```python
from build123d import *

# Parameters (mm, degrees)
F1_DEPTH = 50.8
F2_SIZE  = 5.08
F3_W     = 6.35
F3_H     = 6.35
F4_DEPTH = 38.1


with BuildPart() as f1:
    # F0 (on Front) → F1 (new body)
    with BuildSketch(Plane.XZ):
        Polygon((12.496759, 6.899342), (0.273374, 14.272182), (-12.223385, 7.37284), (-12.496759, -6.899342), (-0.273374, -14.272182), (12.223385, -7.37284), align=None)
    extrude(amount=F1_DEPTH)

    # F2
    f2_edges = [f1.edges().sort_by_distance(p)[0] for p in [
        (6.385067, 0, 10.585762),
        (12.360072, 0, -0.236749),
        (5.975005, 0, -10.822511),
        (-6.385067, 0, -10.585762),
        (-12.360072, 0, 0.236749),
        (-5.975005, 0, 10.822511),
    ]]
    chamfer(f2_edges, length=F2_SIZE)

    # F3 (on face) → F4 (cut)
    with BuildSketch(Plane(origin=(0, 0, 0), x_dir=(-1, 0, 0), z_dir=(0, 1, 0))):
        Rectangle(F3_W, F3_H)
    extrude(amount=-F4_DEPTH, mode=Mode.SUBTRACT)


solid = f1.part
```
The model under review builds one solid part; all positions refer to its coordinate system, in mm. A direction names the side the tool comes from. Coordinates: 2 decimals unless noted, no trailing zeros. Order: outer loops, then holes, each group sorted by start corner. A loop starts at its lowest first (then second) coordinate and runs counter-clockwise, first axis right, second up. Notation, with made-up numbers: (16.5, -39) -> (65.5, -39) arc R24 ccw to (65.5, -27) -> close; hole circle Ø2 at (74, 72). An arc over 180 degrees is marked (long way). Answer in a Markdown table with one row per item. Add a question column.
Item 1: To check wall thickness, follow probe 1 along Y at (x, z) = (-2.5, -2); probe 2 along Z at (x, y) = (0.5, -22.5) (3 decimals); probe 3 along Z at (x, y) = (-1.5, -25) (3 decimals). State the ranges of each line that lie inside material, in increasing order.
Item 2: Mouldability with a two-part tool opening along Z and no side actions: class faces 1 (the flat face through (3.175, -19, 0)), 2 (the flat face through (-3.175, -19, 0)), 3 (the flat face through (-5.89, -27.62, 10.87)), 4 (the flat face through (-6.471, -27.62, -10.534)) as +Z half, -Z half, draft (parallel to the pull), parting line (faces both ways), or undercut.
Item 3: We need section A-A on y = -29. Write out the cut boundary in (x, z) (3 decimals).
Item 4: Clearance check with flat-ended pins moving along their axes: pin 1 (3 mm diameter, centred on x = -0.5, y = -28, fed in from -Z); pin 2 (1.5 mm diameter, centred on y = -43.5, z = 10.5, fed in from +X); pin 3 (7 mm diameter, centred on y = -18.5, z = 0, fed in from +X); pin 4 (3 mm diameter, centred on x = 3, y = -31.5, fed in from +Z). State where each tip first meets the part, or that it passes through.
Item 5: Machinability: for faces 5 (the flat face through (0, -50.8, 0)), 6 (the flat face through (0, -38.1, 0)), which of the approach directions +Z, -Z, +X, -X, +Y, -Y give a long, thin tool a straight path to every point of the face, cutting with its end or side? Answer none if there is none.
Item 6: We need section C-C on y = -45. Write out the cut boundary in (x, z), plus the area to 3 significant figures.
Item 7: We need section B-B on z = -1.5. Write out the cut boundary in (x, y) (3 decimals).
Item 8: We need section D-D on x = 4. Write out the cut boundary in (y, z), plus the area to 3 significant figures.
Final values:
| question | item | result |
|---|---|---|
| 1 | probe 1 | y = -50.8 to -38.1 |
| 1 | probe 2 | z = -13.845 to -3.175, 3.175 to 14.135 |
| 1 | probe 3 | z = -13.532 to -3.175, 3.175 to 13.293 |
| 2 | face 1 | undercut |
| 2 | face 2 | undercut |
| 2 | face 3 | +Z half |
| 2 | face 4 | -Z half |
| 3 | outline | (-12.497, -6.899) -> (-0.273, -14.272) -> (12.223, -7.373) -> (12.497, 6.899) -> (0.273, 14.272) -> (-12.223, 7.373) -> close; hole (-3.175, -3.175) -> (3.175, -3.175) -> (3.175, 3.175) -> (-3.175, 3.175) -> close |
| 4 | pin 1 | stops at z = -14.27 |
| 4 | pin 2 | stops at x = 7.77 |
| 4 | pin 3 | stops at x = 12.43 |
| 4 | pin 4 | stops at z = 13.53 |
| 5 | face 5 | +Z, -Z, +X, -X, -Y |
| 5 | face 6 | +Y |
| 6 | outline | (-12.5, -6.9) -> (-0.27, -14.27) -> (12.22, -7.37) -> (12.5, 6.9) -> (0.27, 14.27) -> (-12.22, 7.37) -> close |
| 6 | area | 529 mm2 |
| 7 | outline | (-12.393, -50.8) -> (12.336, -50.8) -> (12.336, -5.08) -> (7.255, 0) -> (3.175, 0) -> (3.175, -38.1) -> (-3.175, -38.1) -> (-3.175, 0) -> (-7.312, 0) -> (-12.393, -5.08) -> close |
| 8 | outline | (-50.8, -11.91) -> (-5.08, -11.91) -> (0, -6.11) -> (0, 6.09) -> (-5.08, 12.02) -> (-50.8, 12.02) -> close |
| 8 | area | 1,190 mm2 |
